Part print with two shaded views. Sizes in mm from the minimum x, y, z corner. A direction names the side the tool comes from. Give positions to 0.01 mm unless a question says otherwise; leave off trailing zeros. Write each loop counter-clockwise with the first axis right and the second up, starting at its lowest first coordinate (ties: lowest second). Pieces come first, ordered by that corner, then holes.
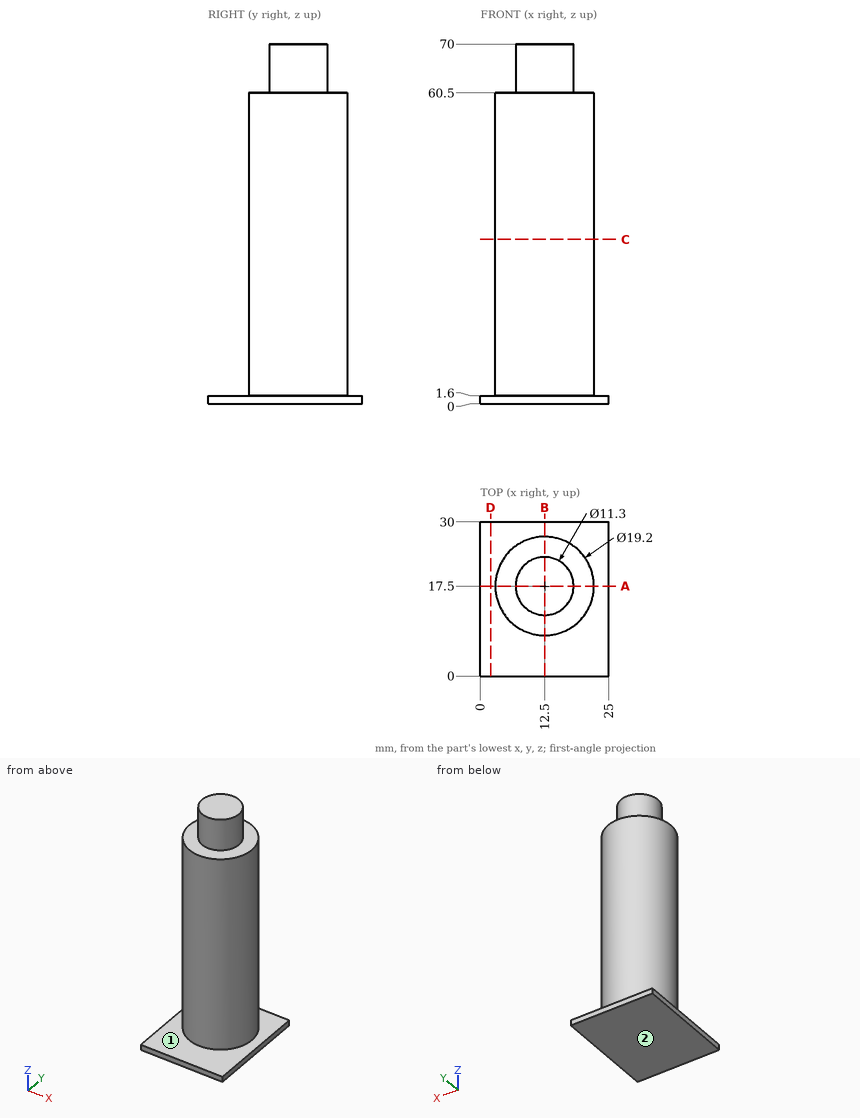
1) Wall check: L1, parallel to Z at x = 22, y = 11; L2, parallel to Z at x = 10.75, y = 25; L3, parallel to X at y = 17, z = 32.5. Give the ranges that are in metal, low to high.
Answers follow:
L1: z = 0 to 1.6
L2: z = 0 to 60.5
L3: x = 2.91 to 22.09
2) Pin check, flat tips, straight feed: pin 1 Ø8 at (y, z) = (25, 15) entering from -X; pin 2 Ø4 at (x, z) = (18, 36.5) entering from +Y; pin 3 Ø1 at (x, z) = (18, 56.5) entering from +Y; pin 4 Ø2 at (y, z) = (5.5, 24.5) entering from +X. Stop position of each tip, or through.
Answers follow:
pin 1: stops at x = 3.56
pin 2: stops at y = 26.44
pin 3: stops at y = 25.7
pin 4: passes through
3) Saw through at D-D, the plane x = 2. Write the cut outline in (y, z), then the cut area to 3 significant figures.
Answers follow:
outline: (0, 0) - (30, 0) - (30, 1.6) - (0, 1.6) - close
area: 48.0 mm2
4) Saw through at B-B, the plane x = 12.5. Write the cut outline in (y, z), then the cut area to 3 significant figures.
Answers follow:
outline: (0, 0) - (30, 0) - (30, 1.6) - (27.1, 1.6) - (27.1, 60.5) - (23.15, 60.5) - (23.15, 70) - (11.85, 70) - (11.85, 60.5) - (7.9, 60.5) - (7.9, 1.6) - (0, 1.6) - close
area: 1,290 mm2
5) Saw through at A-A, the plane y = 17.5. Write the cut outline in (x, z).
Answers follow:
outline: (0, 0) - (25, 0) - (25, 1.6) - (22.1, 1.6) - (22.1, 60.5) - (18.15, 60.5) - (18.15, 70) - (6.85, 70) - (6.85, 60.5) - (2.9, 60.5) - (2.9, 1.6) - (0, 1.6) - close
6) 3-axis set-ups, long thin cutter, end or side, ignore diameter. For the marked faces 1 and 2: which of +Z, -Z, +X, -X, +Y, -Y reach the whole face in a straight line?
Answers follow:
face 1: +Z
face 2: -Z, +X, -X, +Y, -Y
7) Saw through at C-C, the plane z = 32. Write the cut outline in (x, y), then the cut area to 3 significant figures.
Answers follow:
outline: circle Ø19.2 at (12.5, 17.5)
area: 290 mm2
